Source: CAD feature listing. Evaluate the final solid. Frame: model axes, mm. A direction names the side the tool comes from. Coordinates: 2 decimals unless noted, no trailing zeros. Order: outer loops, then holes, each group sorted by start corner. A loop starts at its lowest first (then second) coordinate and runs counter-clockwise, first axis right, second up.
```python
from build123d import *

# Parameters (mm, degrees)
CROQUIS1_R              = 11
SALIENTE_EXTRUIR1_DEPTH = 13
CROQUIS2_R              = 8
CORTAR_EXTRUIR1_DEPTH   = 5
CROQUIS3_R              = 1.5
CORTAR_EXTRUIR2_DEPTH   = 15
CROQUIS4_R              = 4
SALIENTE_EXTRUIR2_DEPTH = 52.8


with BuildPart() as part:
    # Croquis1 → Saliente-Extruir1 (new body)
    with BuildSketch(Plane.XY):
        Circle(CROQUIS1_R)
    extrude(amount=SALIENTE_EXTRUIR1_DEPTH)

    # Croquis2 → Cortar-Extruir1 (cut)
    with BuildSketch(Plane.XY.offset(13)):
        Circle(CROQUIS2_R)
    extrude(amount=-CORTAR_EXTRUIR1_DEPTH, mode=Mode.SUBTRACT)

    # Croquis3 → Cortar-Extruir2 (cut)
    with BuildSketch(Plane(origin=(0, 0, 0), x_dir=(0, 0, -1), z_dir=(1, 0, 0))):
        with Locations((-5, 0)):
            Circle(CROQUIS3_R)
    extrude(amount=-CORTAR_EXTRUIR2_DEPTH, mode=Mode.SUBTRACT)

    # Croquis4 → Saliente-Extruir2 (add)
    with BuildSketch(Plane(origin=(0, 0, 0), x_dir=(-1, 0, 0), z_dir=(0, 0, -1))):
        Circle(CROQUIS4_R)
    extrude(amount=SALIENTE_EXTRUIR2_DEPTH)


solid = part.part
```
Q1. Section query B-B on y = 0. Output: boundary loops of the cut face in (x, z), plus the area to 3 significant figures.
Solutions:
outline: (-11, 0) - (-4, 0) - (-4, -52.8) - (4, -52.8) - (4, 0) - (11, 0) - (11, 13) - (8, 13) - (8, 8) - (-8, 8) - (-8, 13) - (-11, 13) - (-11, 6.5) - (0, 6.5) - (0, 3.5) - (-11, 3.5) - close
area: 595 mm2
Q2. Section query A-A on x = -1. Output: boundary loops of the cut face in (y, z), plus the area to 3 significant figures.
Solutions:
outline: (-10.95, 0) - (-3.87, 0) - (-3.87, -52.8) - (3.87, -52.8) - (3.87, 0) - (10.95, 0) - (10.95, 13) - (7.94, 13) - (7.94, 8) - (-7.94, 8) - (-7.94, 13) - (-10.95, 13) - close; hole circle Ø3 at (0, 5)
area: 607 mm2
Q3. Section query D-D on z = -3. Output: boundary loops of the cut face in (x, y).
Solutions:
outline: circle Ø8 at (0, 0)
Q4. Material intervals for line 1 along Z through (x, y) = (-2.25, 0); line 2 along Y through (x, z) = (0, 11.95); line 3 along Z through (x, y) = (0.5, 4.75), sorted ascending.
Solutions:
line 1: z = -52.8 to 3.5, 6.5 to 8
line 2: y = -11 to -8, 8 to 11
line 3: z = 0 to 8
Q5. Pull-direction query (Z, two-part tool) for faces 1 (the cylindrical face through (-1.73, -7.81, 10.54)), 2 (the flat face through (0, 0, 5)), 3 (the flat face through (0, -5, 0)); classes: pulls with the +Z half, pulls with the -Z half, needs draft (parallel to the pull), parting line crosses it, or undercut.
Solutions:
face 1: needs draft
face 2: undercut
face 3: pulls with the -Z half
Q6. Set-up query: faces 4 (the cylindrical face through (10.161, -4.213, 6.409)), 5 (the flat face through (0, 0, 8)), 6 (the cylindrical face through (0.867, -3.905, -26.03)), 7 (the cylindrical face through (-5.4, -0.9, 6.2)), 8 (the flat face through (-2, -8, 13)). Return all of +Z, -Z, +X, -X, +Y, -Y with unobstructed straight access to the full face (end or side cutting, diameter ignored); none if empty.
Solutions:
face 4: +Z, -Z
face 5: +Z
face 6: -Z
face 7: -X
face 8: +Z, +X, -X, +Y, -Y
Q7. Pin query (flat end, axial travel): P1, Ø1.5, axis at x = 2.5, y = -8, coming from the -Z side; P2, Ø4, axis at y = 2.5, z = -13, coming from the -X side; P3, Ø8, axis at x = -4, z = -4.5, coming from the +Y side. Return the tip coordinate at first contact, or that it passes through.
Solutions:
P1: stops at z = 0
P2: stops at x = -3.97
P3: stops at y = 4
Q8. Section query C-C on x = 5.25. Output: boundary loops of the cut face in (y, z), plus the area to 3 significant figures.
Solutions:
outline: (-9.67, 0) - (9.67, 0) - (9.67, 13) - (6.04, 13) - (6.04, 8) - (-6.04, 8) - (-6.04, 13) - (-9.67, 13) - close
area: 191 mm2
